Autodesk Inventor part; units mm, degrees
ref_plane "YZ Plane" through (0, 0, 0) normal (1, 0, 0) x (0, 1, 0)
ref_plane "XZ Plane" through (0, 0, 0) normal (0, 1, 0) x (-1, 0, 0)
ref_plane "XY Plane" through (0, 0, 0) normal (0, 0, 1) x (1, 0, 0)
sketch "Sketch1" plane through (0, 0, 0) normal (0, 1, 0) x (-1, 0, 0)
  circle A0 centre (0, 0) radius 10.922
  arc A1 (0, 15.875) -> (0, -15.875) centre (0, 0) ccw
  line L0 (0, 0) -> (36.703, 0) construction
  arc A2 (36.703, -6.35) -> (36.703, 6.35) centre (36.703, 0) ccw
  line L1 (0, 15.875) -> (36.703, 6.35)
  line L2 (0, -15.875) -> (36.703, -6.35)
  circle A3 centre (36.703, 0) radius 1.3335
  dimension "d0" = 21.844
  dimension "d1" = 31.75
  dimension "d2" = 36.703
  dimension "d3" = 12.7
  dimension "d4" = 2.667
extrude "Extrusion1" add sketch "Sketch1" along normal blind 4.572
properties part number "Light_Hooker"
Verification items for the finished model (mm, model axes). Coordinates: 2 decimals unless noted, no trailing zeros. Write each loop counter-clockwise with the first axis right and the second up, starting at its lowest first coordinate (ties: lowest second). Pieces come first, ordered by that corner, then holes. Notation, with made-up numbers: (81, 54) -> (120, 54) arc R8 cw to (120, 65) -> close; hole circle Ø11 at (-28, -6.75). An arc over 180 degrees is marked (long way). One line per item, written item: value. Start each with the question number.
Q1. Mould release check, pull along Z, two halves, no side actions. Record for faces 1 (the cylindrical face through (-10.418, 2.254, -3.281)), 2 (the flat face through (-18.09, 2.25, -11.18)), 3 (the cylindrical face through (-43.05, 2.25, 0.14)): pulls with the +Z half, pulls with the -Z half, needs draft (parallel to the pull), parting line crosses it, or undercut.
Q2. Cross-section at D-D on z = -4. Enter the section's corners in (x, y), and give its area (3 significant figures).
Q3. Cross-section at A-A on z = 0. Enter the section's corners in (x, y) (1 decimal).
Q4. Cross-section at B-B on y = 3.6. State how many separate pieces and enclosed holes the cut face has, and give its area (3 significant figures).
Q5. Thickness scan on L1, parallel to Z at x = 0, y = 1.9 (3 decimals); L2, parallel to Z at x = -4, y = 4.45; L3, parallel to X at y = 2.65, z = 4. Record the ranges inside material, lowest first. Write a range as from..to.
Q6. Go/stop test with flat-tipped pins: P1, Ø2, axis at x = 6.5, y = 1.5, coming from the +Z side; P2, Ø2, axis at x = -34.5, y = 1, coming from the +Z side; P3, Ø1, axis at x = -22.5, y = 1, coming from the -Z side. Record where each tip stops, or that it passes through.
Q7. Cross-section at C-C on x = 10. Enter the section's corners in (y, z), and give its area (3 significant figures).
Checked values:
1. face 1: undercut
1. face 2: pulls with the -Z half
1. face 3: parting line crosses it
2. outline: (-41.63, 0) -> (-10.16, 0) -> (-10.16, 4.57) -> (-41.63, 4.57) -> close; (10.16, 0) -> (15.36, 0) -> (15.36, 4.57) -> (10.16, 4.57) -> close
2. area: 168 mm²
3. outline: (-43.1, 0) -> (-38, 0) -> (-38, 4.6) -> (-43.1, 4.6) -> close; (-35.4, 0) -> (-10.9, 0) -> (-10.9, 4.6) -> (-35.4, 4.6) -> close; (10.9, 0) -> (15.9, 0) -> (15.9, 4.6) -> (10.9, 4.6) -> close
4. separate pieces: 1
4. enclosed holes: 2
4. area: 895 mm²
5. L1: z = -15.875..-10.922, 10.922..15.875
5. L2: z = -14.84..-10.16, 10.16..14.84
5. L3: x = -41.63..-10.16, 10.16..15.36
6. P1: stops at z = 14.89
6. P2: stops at z = 7.18
6. P3: stops at z = -10.17
7. outline: (0, -12.33) -> (4.57, -12.33) -> (4.57, -4.39) -> (0, -4.39) -> close; (0, 4.39) -> (4.57, 4.39) -> (4.57, 12.33) -> (0, 12.33) -> close
7. area: 72.6 mm²
